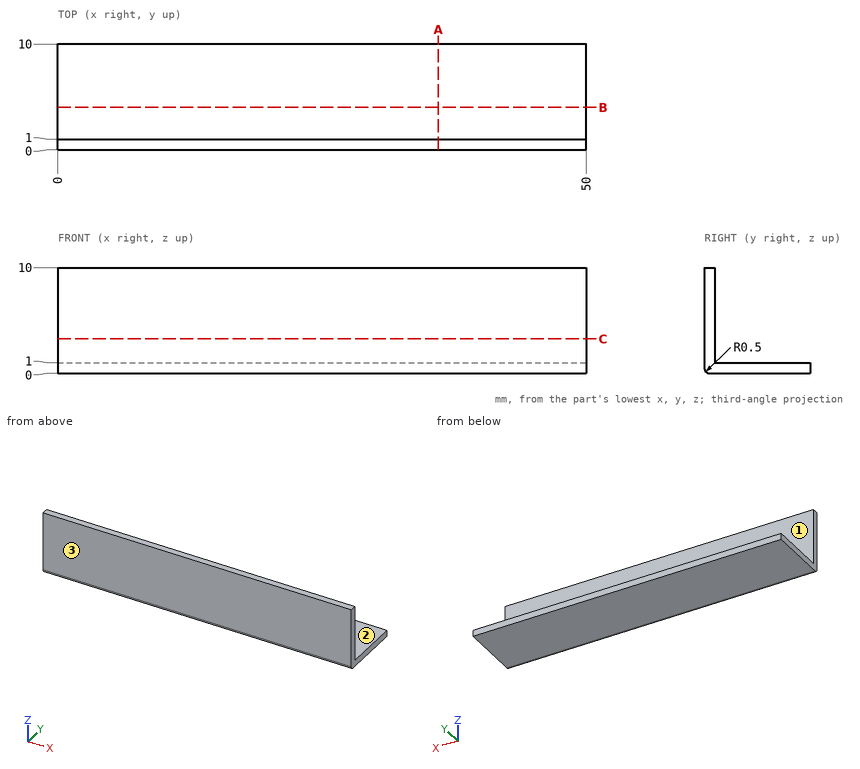
The figure shows three views and two pictorial views of one solid part (mm, origin at its lowest corner). Answer the questions. Coordinates: 2 decimals unless noted, no trailing zeros. Write each loop counter-clockwise with the first axis right and the second up, starting at its lowest first coordinate (ties: lowest second). Pieces come first, ordered by that corner, then holes. Notation, with made-up numbers: (-14, 68.25) -> (26, 68.25) arc R33 ccw to (26, 101.25) -> close; hole circle Ø9 at (-30, -27). An arc over 180 degrees is marked (long way). Answer as a JSON object with one key per item and string values.
Q1. A flat-ended cylindrical pin translates along its axis: pin 1 Ø2.5 at (x, y) = (30.5, 6.5) entering from +Z. Find the tip coordinate at first contact, or state that the pin passes through.
The answers:
{"pin 1": "stops at z = 1"}
Q2. The part is cut by section A-A on x = 36. Give the vertices of the cut face in (y, z), then the cut area to 3 significant figures.
The answers:
{"outline": "(0, 0.5) arc R0.5 ccw to (0.5, 0) -> (10, 0) -> (10, 1) -> (1, 1) -> (1, 10) -> (0, 10) -> close", "area": "18.9 mm2"}
Q3. Determine the mould class of the marked faces 1, 2 and 3 for opening direction Y: pulls with the +Y half, pulls with the -Y half, needs draft (parallel to the pull), parting line crosses it, or undercut.
The answers:
{"face 1": "pulls with the +Y half", "face 2": "needs draft", "face 3": "pulls with the -Y half"}
Q4. The part is cut by section B-B on y = 4. Give the vertices of the cut face in (x, z), then the cut area to 3 significant figures.
The answers:
{"outline": "(0, 0) -> (50, 0) -> (50, 1) -> (0, 1) -> close", "area": "50.0 mm2"}
Q5. Consider line 1 (Z direction, x = 12, y = 5). Determine where the line is inside the solid, lowest interval first. Write a range as [from, to].
The answers:
{"line 1": "z = [0, 1]"}
